Work out the finished part from the listing and answer in its coordinate system (mm). Face numbers are marked on the shaded views. A direction names the side the tool comes from. Round coordinates to 2 decimals unless told otherwise and drop trailing zeros. Loops run counter-clockwise (first coordinate to the right, second up) from the corner with the lowest first, then second, coordinate; pieces in that order, holes last.
from build123d import *

# Parameters (mm, degrees)
CROQUIS1_W              = 25
CROQUIS1_H              = 34
SALIENTE_EXTRUIR1_DEPTH = 6
CROQUIS2_W              = 7
CROQUIS2_H              = 5
SALIENTE_EXTRUIR2_DEPTH = 6
CORTAR_EXTRUIR1_REACH   = 44.626
CROQUIS3_W              = 11
CROQUIS3_H              = 26
REDONDEO1_R             = 4
SALIENTE_EXTRUIR3_DEPTH = 12
SALIENTE_EXTRUIR4_DEPTH = 2
CORTAR_EXTRUIR2_REACH   = 70.45
CROQUIS7_R              = 1.75
CORTAR_EXTRUIR3_REACH   = 67.577
CROQUIS8_W              = 27.3
CROQUIS8_H              = 5
SALIENTE_EXTRUIR5_DEPTH = 6


with BuildPart() as part:
    # Croquis1 → Saliente-Extruir1 (new body)
    with BuildSketch(Plane.XY):
        with Locations((-12.5, -17)):
            Rectangle(CROQUIS1_W, CROQUIS1_H)
    extrude(amount=SALIENTE_EXTRUIR1_DEPTH)

    # Croquis2 → Saliente-Extruir2 (add)
    with BuildSketch(Plane.XY.offset(6)):
        with Locations((-21.5, -5.5)):
            Rectangle(CROQUIS2_W, CROQUIS2_H)
        with Locations((-3.5, -5.5)):
            Rectangle(CROQUIS2_W, CROQUIS2_H)
        with Locations((-3.5, -31.5)):
            Rectangle(CROQUIS2_W, CROQUIS2_H)
        with Locations((-21.5, -31.5)):
            Rectangle(CROQUIS2_W, CROQUIS2_H)
    extrude(amount=SALIENTE_EXTRUIR2_DEPTH)

    # Croquis3 → Cortar-Extruir1 (cut, up to next)
    with BuildSketch(Plane.XY.offset(6), mode=Mode.PRIVATE) as cortar_extruir1_sk1:
        with Locations((-12.5, -16)):
            Rectangle(CROQUIS3_W, CROQUIS3_H)
    cortar_extruir1_tool1 = extrude(cortar_extruir1_sk1.sketch, amount=-CORTAR_EXTRUIR1_REACH, mode=Mode.PRIVATE) & part.part
    add(cortar_extruir1_tool1.solids().sort_by_distance((-12.5, -16, 6))[0], mode=Mode.SUBTRACT)

    # Redondeo1
    # the kernel refuses this fillet: 4 mm, written as the material it adds along each edge
    with BuildSketch(Plane(origin=(-18, -29, 6), x_dir=(0, 1, 0), z_dir=(0, 0, -1)), Plane(origin=(-7, -29, 6), x_dir=(-1, 0, 0), z_dir=(0, 0, -1)), Plane(origin=(-18, -3, 6), x_dir=(1, 0, 0), z_dir=(0, 0, -1))) as redondeo1_piece_1:
        with BuildLine():
            CenterArc((REDONDEO1_R, REDONDEO1_R), REDONDEO1_R, 180, 90)
            Line((0, REDONDEO1_R), (0, 0))
            Line((0, 0), (REDONDEO1_R, 0))
        make_face()
    extrude(amount=6)
    with BuildSketch(Plane(origin=(-7, -3, 6), x_dir=(-1, 0, 0), z_dir=(0, 0, -1))) as redondeo1_piece_2:
        with BuildLine():
            CenterArc((REDONDEO1_R, -REDONDEO1_R), REDONDEO1_R, 90, 90)
            Line((0, -REDONDEO1_R), (0, 0))
            Line((0, 0), (REDONDEO1_R, 0))
        make_face()
    extrude(amount=6)
    # the kernel refuses this fillet: 4 mm, written as the material it takes off along each edge
    with BuildSketch(Plane(origin=(0, 0, -10), x_dir=(-1, 0, 0), z_dir=(0, 0, 1))) as redondeo1_2_piece_1:
        with BuildLine():
            CenterArc((REDONDEO1_R, REDONDEO1_R), REDONDEO1_R, 180, 90)
            Line((0, REDONDEO1_R), (0, 0))
            Line((0, 0), (REDONDEO1_R, 0))
        make_face()
    extrude(amount=26, mode=Mode.SUBTRACT)
    with BuildSketch(Plane(origin=(0, -34, 22), x_dir=(0, 1, 0), z_dir=(0, 0, -1)), Plane(origin=(-25, -34, -10), x_dir=(0, 1, 0), z_dir=(0, 0, 1))) as redondeo1_2_piece_2:
        with BuildLine():
            CenterArc((REDONDEO1_R, -REDONDEO1_R), REDONDEO1_R, 90, 90)
            Line((0, -REDONDEO1_R), (0, 0))
            Line((0, 0), (REDONDEO1_R, 0))
        make_face()
    extrude(amount=32, mode=Mode.SUBTRACT)
    with BuildSketch(Plane(origin=(-25, 0, -10), x_dir=(1, 0, 0), z_dir=(0, 0, 1))) as redondeo1_2_piece_3:
        with BuildLine():
            CenterArc((REDONDEO1_R, -REDONDEO1_R), REDONDEO1_R, 90, 90)
            Line((0, -REDONDEO1_R), (0, 0))
            Line((0, 0), (REDONDEO1_R, 0))
        make_face()
    extrude(amount=26, mode=Mode.SUBTRACT)

    # Croquis5 → Saliente-Extruir3 (add)
    with BuildSketch(Plane(origin=(0, 0, 0), x_dir=(-1, 0, 0), z_dir=(0, 0, -1))):
        with BuildLine():
            Line((25, -29), (25, -30))
            ThreePointArc((25, -30), (23.828427125, -32.828427125), (21, -34))
            Line((21, -34), (25, -34))
            Line((25, -34), (59.4, -34))
            Line((59.4, -34), (59.4, -24))
            Line((59.4, -24), (25, -24))
            Line((25, -24), (25, -29))
        make_face()
    extrude(amount=-SALIENTE_EXTRUIR3_DEPTH)

    # Croquis6 → Saliente-Extruir4 (add)
    with BuildSketch(Plane.XY.offset(12)):
        Polygon((-18, -29), (-25, -29), (-25, -24), (-59.4, -24), (-59.4, -34), (-18, -34), align=None)
    extrude(amount=SALIENTE_EXTRUIR4_DEPTH)

    # Cortar-Extruir2: up to this face of the body (flat: up to its plane)
    cortar_extruir2_end = Plane(part.part.faces().sort_by_distance((-34.409507042, -34, 6.559859155))[0])
    # Croquis7 → Cortar-Extruir2 (cut, up to the picked face)
    with BuildSketch(Plane(origin=(0, -3, 0), x_dir=(1, 0, 0), z_dir=(0, 1, 0)), mode=Mode.PRIVATE) as cortar_extruir2_sk1:
        with Locations(Location((-21.772983346, -9, 0), (0, 0, 270))):
            Circle(CROQUIS7_R)
    cortar_extruir2_tool1 = split(extrude(cortar_extruir2_sk1.sketch, amount=-CORTAR_EXTRUIR2_REACH, mode=Mode.PRIVATE), bisect_by=cortar_extruir2_end, keep=Keep.BOTH, mode=Mode.PRIVATE)
    # Croquis7 → Cortar-Extruir2 (cut, up to the picked face)
    with BuildSketch(Plane(origin=(0, -3, 0), x_dir=(1, 0, 0), z_dir=(0, 1, 0)), mode=Mode.PRIVATE) as cortar_extruir2_sk2:
        with Locations(Location((-3.227016654, -9, 0), (0, 0, 243.787297197))):
            Circle(CROQUIS7_R)
    cortar_extruir2_tool2 = split(extrude(cortar_extruir2_sk2.sketch, amount=-CORTAR_EXTRUIR2_REACH, mode=Mode.PRIVATE), bisect_by=cortar_extruir2_end, keep=Keep.BOTH, mode=Mode.PRIVATE)
    add(cortar_extruir2_tool1.solids().sort_by(Axis((-21.772983, -3, 9), (0, -1, 0)))[0], mode=Mode.SUBTRACT)
    add(cortar_extruir2_tool2.solids().sort_by(Axis((-3.227017, -3, 9), (0, -1, 0)))[0], mode=Mode.SUBTRACT)

    # Croquis8 → Cortar-Extruir3 (cut, up to next)
    with BuildSketch(Plane(origin=(0, -24, 0), x_dir=(1, 0, 0), z_dir=(0, 1, 0)), mode=Mode.PRIVATE) as cortar_extruir3_sk1:
        with Locations((-42.2, -7)):
            Rectangle(CROQUIS8_W, CROQUIS8_H)
    cortar_extruir3_tool1 = extrude(cortar_extruir3_sk1.sketch, amount=-CORTAR_EXTRUIR3_REACH, mode=Mode.PRIVATE) & part.part
    add(cortar_extruir3_tool1.solids().sort_by_distance((-42.2, -24, 7))[0], mode=Mode.SUBTRACT)

    # Croquis9 → Saliente-Extruir5 (add)
    with BuildSketch(Plane(origin=(0, 0, 0), x_dir=(-1, 0, 0), z_dir=(0, 0, -1))):
        Polygon((2.0503268, -0.507325607), (25, -13.757325607), (23.5, -16.355401819), (17.437822174, -12.855401819), (6.612504626, -6.605401819), (0.5503268, -3.105401819), align=None)
        Polygon((25.33358423, -36.281262865), (2.38391103, -49.531262865), (0.5503268, -46.355401819), (6.612504626, -42.855401819), (17.437822174, -36.605401819), (23.5, -33.105401819), align=None)
    extrude(amount=SALIENTE_EXTRUIR5_DEPTH)


solid = part.part
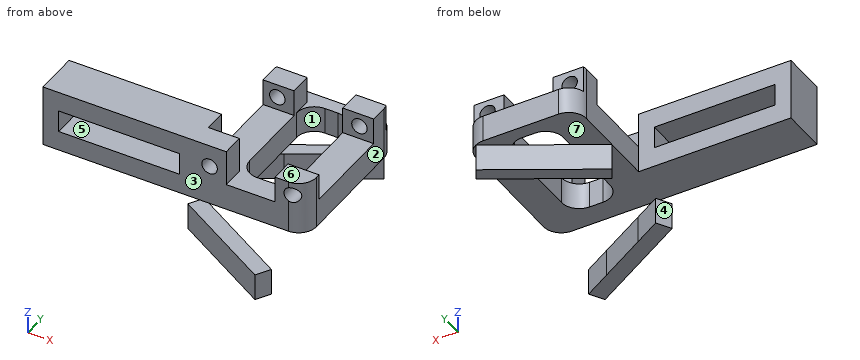
Item 1: Section D-D, the plane x = -12 is taken. Give the vertices of the cut face in (y, z), plus the area to 3 significant figures.
Item 2: Section A-A, the plane x = -44 is taken. Give the vertices of the cut face in (y, z), plus the area to 3 significant figures.
Item 3: Each of these flat-tipped pins is pushed along its axis until it touches: P1, Ø1.8, axis at x = -22, z = 9.5, coming from the -Y side; P2, Ø6, axis at y = -13, z = 3, coming from the -X side; P3, Ø16.5, axis at x = -28.5, y = -23.5, coming from the -Z side; P4, Ø4.5, axis at x = -15, y = -7, coming from the +Z side. Where does it stop, or does it pass through?
Item 4: Section B-B, the plane y = -5 is taken. Give the vertices of the cut face in (x, z).
Item 5: Straight lines are drawn through the part: line 1 (X direction, y = -25, z = 5.25); line 2 (X direction, y = -25, z = 9.25); line 3 (X direction, y = -9.5, z = 2). For each, find the intervals that lie inside material, in ascending order.
Item 6: Determine the mould class of the marked faces 1, 2 and 3 for opening direction X: pulls with the +X half, pulls with the -X half, needs draft (parallel to the pull), parting line crosses it, or undercut.
Item 7: For the marked faces 4, 5, 6 and 7, determine the directions among +Z, -Z, +X, -X, +Y, -Y from which every point of the face is accessible in a straight line to the end or side of a thin tool.
Item 8: Section C-C, the plane z = 2 is taken. Give the vertices of the cut face in (x, y), plus the area to 3 significant figures.
Answer below:
1. outline: (-43.98, -6) - (-39.74, -6) - (-39.74, 0) - (-43.98, 0) - close; (-34, 0) - (-29, 0) - (-29, 6) - (-34, 6) - close; (-9.72, -6) - (-6.25, -6) - (-6.25, 0) - (-9.72, 0) - close; (-3, 0) - (0, 0) - (0, 6) - (-3, 6) - close
1. area: 94.2 mm2
2. outline: (-34, 0) - (-24, 0) - (-24, 4.5) - (-34, 4.5) - close; (-34, 9.5) - (-24, 9.5) - (-24, 14) - (-34, 14) - close
2. area: 90.0 mm2
3. P1: passes through
3. P2: stops at x = -25
3. P3: stops at z = 0
3. P4: stops at z = 0
4. outline: (-25, 0) - (-17.46, 0) - (-17.46, 6) - (-18, 6) - (-18, 12) - (-25, 12) - close; (-9.83, -6) - (-3.83, -6) - (-3.83, 0) - (0, 0) - (0, 12) - (-7, 12) - (-7, 6) - (-7.54, 6) - (-7.54, 0) - (-9.83, 0) - close; hole circle Ø3.5 at (-21.77, 9); hole circle Ø3.5 at (-3.23, 9)
5. line 1: x = -59.4 to -55.85, -28.55 to -18, -7 to 0
5. line 2: x = -59.4 to -55.85, -28.55 to -25
5. line 3: x = -25 to -18, -7 to 0
6. face 1: undercut
6. face 2: pulls with the +X half
6. face 3: needs draft
7. face 4: -Z, -X
7. face 5: +Y, -Y
7. face 6: +Z, +X, +Y, -Y
7. face 7: -Z, -X, +Y
8. outline: (-59.4, -34) - (-4, -34) arc R4 ccw to (0, -30) - (0, -4) arc R4 ccw to (-4, 0) - (-21, 0) arc R4 ccw to (-25, -4) - (-25, -24) - (-59.4, -24) - close; hole (-18, -25) arc R4 ccw to (-14, -29) - (-11, -29) arc R4 ccw to (-7, -25) - (-7, -7) arc R4 ccw to (-11, -3) - (-14, -3) arc R4 ccw to (-18, -7) - close
8. area: 911 mm2
